from build123d import *

# Parameters (mm, degrees)
F1_DEPTH = 101.6
F2_T     = -2.54


with BuildPart() as f1:
    # F0 (on Front) → F1 (new body)
    with BuildSketch(Plane.XZ):
        Polygon((91.702374, -0.963147), (-45.017077, 79.898159), (-46.685297, -78.935012), align=None)
    extrude(amount=F1_DEPTH)

    # F2
    f2_openings = [f1.faces().sort_by_distance(p)[0] for p in [
        (-45.851187, -50.8, 0.481574),
    ]]
    offset(amount=F2_T, openings=f2_openings)


solid = f1.part
Geometry check sheet. Reference: the model listing, model coordinates, mm. A direction names the side the tool comes from. Give positions to 0.01 mm unless a question says otherwise; leave off trailing zeros. Loops run counter-clockwise (first coordinate to the right, second up) from the corner with the lowest first, then second, coordinate; pieces in that order, holes last.
(1) Set-up check for faces 4 (the flat face through (21.54, -50.089, -40.495)), 5 (the flat face through (21.71, -50.12, 37.48)): record each of +Z, -Z, +X, -X, +Y, -Y from which the full face is reachable in a straight line by a thin tool's end or side.
From the geometry:
face 4: -Z, +X, +Y, -Y
face 5: -X
(2) Thickness scan on L1, parallel to Y at x = -38.5, z = 30; L2, parallel to Z at x = -26, y = -23.5; L3, parallel to Z at x = 56.5, y = -84. Record the ranges inside material, lowest first.
From the geometry:
L1: y = -101.6 to -99.06, -2.54 to 0
L2: z = -67.28 to -64.36, 65.7 to 68.65
L3: z = -20.8 to -17.88, 16.91 to 19.86
(3) Section check C-C on z = 14.5. Record the cut outline in (x, y), then the cut area to 3 significant figures.
From the geometry:
outline: (-45.7, -101.6) - (65.56, -101.6) - (65.56, 0) - (-45.7, 0) - (-45.7, -2.54) - (60.57, -2.54) - (60.57, -99.06) - (-45.7, -99.06) - close
area: 1,050 mm2
(4) Depth check by flat-ended pin: pin 1 Ø3 at (y, z) = (-74, -60) entering from +X; pin 2 Ø2 at (x, y) = (25, -41.5) entering from -Z; pin 3 Ø8 at (x, y) = (23.5, -16) entering from -Z; pin 4 Ø3 at (x, z) = (-14, 35) entering from +Y. Enter the tip coordinate at first touch or a pass-through.
From the geometry:
pin 1: stops at x = -10.42
pin 2: stops at z = -39.11
pin 3: stops at z = -41.64
pin 4: stops at y = 0
(5) Section check D-D on x = -5. Record the cut outline in (y, z).
From the geometry:
outline: (-101.6, -55.45) - (0, -55.45) - (0, 56.23) - (-101.6, 56.23) - close; hole (-99.06, -52.53) - (-2.54, -52.53) - (-2.54, 53.28) - (-99.06, 53.28) - close
(6) Section check A-A on x = 22.5. Record the cut outline in (y, z), then the cut area to 3 significant figures.
From the geometry:
outline: (-101.6, -39.95) - (0, -39.95) - (0, 39.97) - (-101.6, 39.97) - close; hole (-99.06, -37.04) - (-2.54, -37.04) - (-2.54, 37.01) - (-99.06, 37.01) - close
area: 972 mm2
(7) Release check for a two-part mould opening along Z. For faces 1 (the flat face through (6, -101.6, 2)), 2 (the flat face through (4, -99.06, 2)), 3 (the flat face through (24.3, -50.1, 38.9)) record: released by +Z, released by -Z, zero draft, split by the parting line, or undercut.
From the geometry:
face 1: zero draft
face 2: undercut
face 3: released by +Z
(8) Section check B-B on y = -8.5. Record the cut outline in (x, z), then the cut area to 3 significant figures.
From the geometry:
outline: (-46.69, -78.94) - (91.7, -0.96) - (-45.02, 79.9) - (-45.05, 76.97) - (86.62, -0.91) - (-46.65, -76) - close
area: 792 mm2
